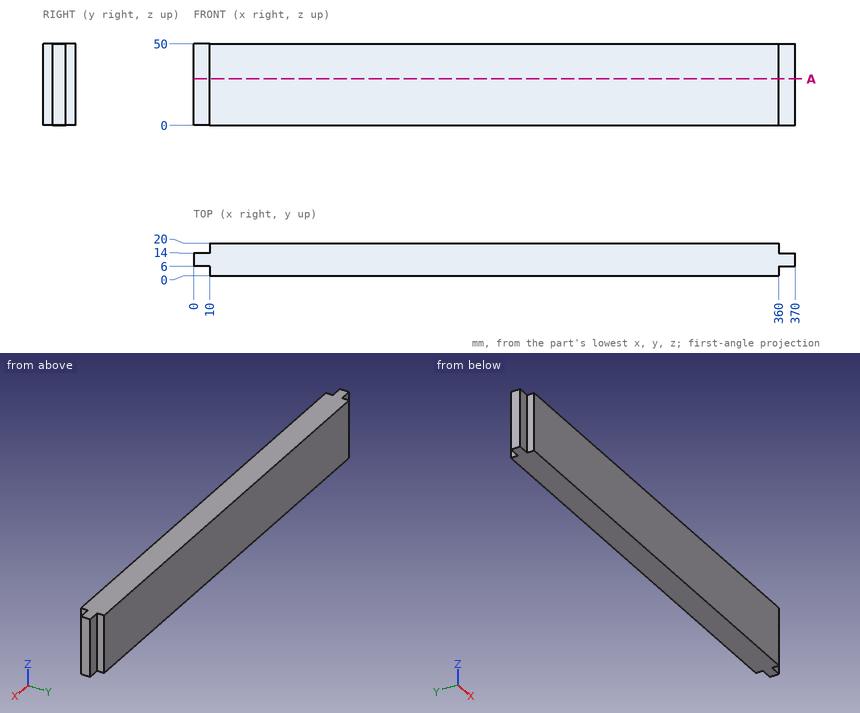
Drawing for the job (mm, zero at the part's lowest x, y, z). Coordinates: 2 decimals unless noted, no trailing zeros. Order: outer loops, then holes, each group sorted by start corner. A loop starts at its lowest first (then second) coordinate and runs counter-clockwise, first axis right, second up. Notation, with made-up numbers: (55, -16) -> (94, -16) arc R14 ccw to (94, 4) -> close; hole circle Ø1 at (38, -35.5). An arc over 180 degrees is marked (long way). One line per item, written item: value.
(1) Probe line 1 (X direction, y = 3, z = 2). List the from-to ranges inside material, lowest first. Write a range as [from, to].
Checked values:
line 1: [10, 360]
(2) Drop flat-ended pins along their axis: pin 1 Ø1.8 at (y, z) = (3, 29.5) entering from +X; pin 2 Ø6.5 at (y, z) = (18, 21) entering from -X; pin 3 Ø3 at (x, z) = (364, 26) entering from -Y. Give the stop position or say it passes through.
Checked values:
pin 1: x = 360
pin 2: x = 10
pin 3: y = 6
(3) Slice it at A-A, the plane z = 28.5. List the corners of the cut face in (x, y), plus the area to 3 significant figures.
Checked values:
outline: (0, 6) -> (10, 6) -> (10, 0) -> (360, 0) -> (360, 6) -> (370, 6) -> (370, 14) -> (360, 14) -> (360, 20) -> (10, 20) -> (10, 14) -> (0, 14) -> close
area: 7,160 mm2
